```python
from build123d import *

# Parameters (mm, degrees)
EXTRUDE_1_DEPTH = 30


with BuildPart() as part:
    # 草图1 → 凸台-拉伸1 (new body)
    with BuildSketch(Plane(origin=(0, 0, 0), x_dir=(1, 0, 0), z_dir=(0, 1, 0))):
        with BuildLine():
            Line((-2.5, 50), (-2.5, 19.843134833))
            ThreePointArc((-2.5, 19.843134833), (-20, 0), (-2.5, -19.843134833))
            Line((-2.5, -19.843134833), (-2.5, -50))
            Line((-2.5, -50), (2.5, -50))
            Line((2.5, -50), (2.5, -19.843134833))
            ThreePointArc((2.5, -19.843134833), (20, 0), (2.5, 19.843134833))
            Line((2.5, 19.843134833), (2.5, 50))
            Line((2.5, 50), (-2.5, 50))
        make_face()
    extrude(amount=EXTRUDE_1_DEPTH)


solid = part.part
```
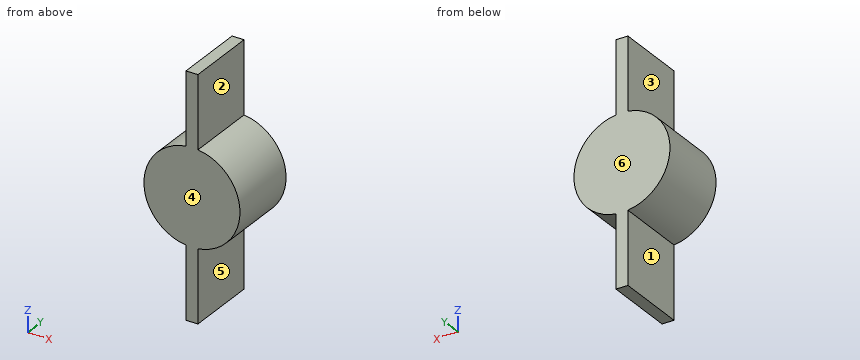
Read the model definition and answer for the solid it produces. Units are mm, in the model's axes. Face numbers are marked on the shaded views. A direction names the side the tool comes from. Coordinates: 2 decimals unless noted, no trailing zeros. Loops run counter-clockwise (first coordinate to the right, second up) from the corner with the lowest first, then second, coordinate; pieces in that order, holes last.
(1) The mould has two halves that part along Y. Classify the marked faces 4, 5 and 6: released by +Y, released by -Y, zero draft, split by the parting line, or undercut.
Solution:
face 4: released by -Y
face 5: zero draft
face 6: released by +Y
(2) The part is cut by section C-C (x = 4). Determine the outline of the cut face in (y, z), and give its area (3 significant figures).
Solution:
outline: (0, -19.6) - (30, -19.6) - (30, 19.6) - (0, 19.6) - close
area: 1,180 mm2
(3) A tool of negligible diameter and unlimited length cuts with its end or side. For the marked faces 1, 2 and 3, from which of +Z, -Z, +X, -X, +Y, -Y can it reach the whole face along a straight path? Write none if from no direction.
Solution:
face 1: -Z, -X, +Y, -Y
face 2: +Z, +X, +Y, -Y
face 3: +Z, -X, +Y, -Y
(4) Flat-ended cylindrical pins translate along their axes: pin 1 Ø4 at (y, z) = (11, 3) entering from +X (3 decimals); pin 2 Ø9 at (y, z) = (10, 28.5) entering from +X; pin 3 Ø5 at (y, z) = (8, 8) entering from +X. Find the tip coordinate at first contact, or state that the pin passes through.
Solution:
pin 1: stops at x = 19.975
pin 2: stops at x = 2.5
pin 3: stops at x = 19.23
(5) The part is cut by section B-B (z = 28). Determine the outline of the cut face in (x, y).
Solution:
outline: (-2.5, 0) - (2.5, 0) - (2.5, 30) - (-2.5, 30) - close
(6) Consider line 1 along X through (y, z) = (2.75, 41.5); line 2 along X through (y, z) = (8, 15.5); line 3 along Z through (x, y) = (4, 16.5). Determine where each line is inside the solid, lowest interval first.
Solution:
line 1: x = -2.5 to 2.5
line 2: x = -12.64 to 12.64
line 3: z = -19.6 to 19.6
(7) The part is cut by section A-A (y = 16). Determine the outline of the cut face in (x, z).
Solution:
outline: (-2.5, -50) - (2.5, -50) - (2.5, -19.84) arc R20 ccw to (2.5, 19.84) - (2.5, 50) - (-2.5, 50) - (-2.5, 19.84) arc R20 ccw to (-2.5, -19.84) - close
